Model file for the job. Use its own axes, mm. Face numbers are marked on the shaded views. A direction names the side the tool comes from. Coordinates: 2 decimals unless noted, no trailing zeros. Loops run counter-clockwise (first coordinate to the right, second up) from the corner with the lowest first, then second, coordinate; pieces in that order, holes last.
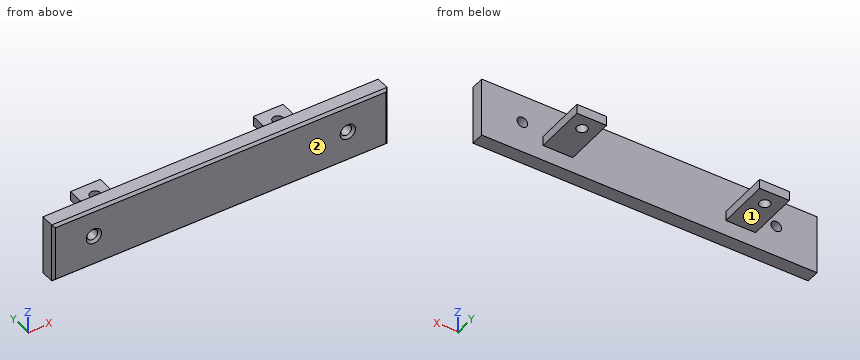
from build123d import *

# Parameters (mm, degrees)
SKETCH059_W             = 140
SKETCH059_H             = 25
SKETCH059_R             = 2.2
PAD026_DEPTH            = 6.5
SKETCH060_W             = 12.4
SKETCH060_H             = 4
PAD027_DEPTH            = 21.5
SKETCH061_R             = 2.2
POCKET032_DEPTH         = 10.609
CHAMFER024_SIZE         = 1
BODY013_ROLL_ANGLE      = 90
BODY013_PLACEMENT_ANGLE = 180


with BuildPart() as part:
    # Sketch059 → Pad026 (new body)
    with BuildSketch(Plane.XY):
        Rectangle(SKETCH059_W, SKETCH059_H)
        with Locations((-53, 0.726)):
            Circle(SKETCH059_R, mode=Mode.SUBTRACT)
        with Locations((53, 0.726)):
            Circle(SKETCH059_R, mode=Mode.SUBTRACT)
    extrude(amount=PAD026_DEPTH)

    # Sketch060 (on Face8 of Pad026) → Pad027 (join)
    with BuildSketch(Plane.XY.offset(6.5)):
        with Locations((-38.154, -3.892)):
            Rectangle(SKETCH060_W, SKETCH060_H)
        with Locations((38.154, -3.892)):
            Rectangle(SKETCH060_W, SKETCH060_H)
    extrude(amount=PAD027_DEPTH)

    # Sketch061 (on Face12 of Pad027) → Pocket032 (cut, through all)
    with BuildSketch(Plane(origin=(0, -1.892, 0), x_dir=(-1, 0, 0), z_dir=(0, 1, 0))):
        with Locations((-38.154, 21.8)):
            Circle(SKETCH061_R)
        with Locations((38.154, 21.8)):
            Circle(SKETCH061_R)
    extrude(amount=-POCKET032_DEPTH, mode=Mode.SUBTRACT)

    # Chamfer024
    chamfer024_edges = [part.edges().sort_by_distance(p)[0] for p in [
        (0, 12.5, 0),
        (70, 0, 0),
        (0, -12.5, 0),
        (-70, 0, 0),
        (50.8, 0.726, 0),
        (-55.2, 0.726, 0),
    ]]
    chamfer(chamfer024_edges, length=CHAMFER024_SIZE)


with BuildPart() as part_1:
    # Body013 roll: moved
    add(part.part.rotate(Axis((0, 0, 0), (1, 0, 0)), BODY013_ROLL_ANGLE))


with BuildPart() as part_2:
    # Body013 placement: moved
    add(part_1.part.moved(Location((0, -145.15, 0))).rotate(Axis((0, -145.15, 0), (0, 0, 1)), BODY013_PLACEMENT_ANGLE))


solid = part_2.part
Q1. Slice it at D-D (x = -19). List the corners of the cut face in (y, z), and give its area (4 significant figures).
Answers:
outline: (-145.15, -11.5) - (-144.15, -12.5) - (-138.65, -12.5) - (-138.65, 12.5) - (-144.15, 12.5) - (-145.15, 11.5) - close
area: 161.5 mm2
Q2. Which spindle directions (+Z, -Z, +X, -X, +Y, -Y) get a long thin tool onto all of the face, cutting with end or side? Do the marked faces 1 and 2. Say none if no direction does.
Answers:
face 1: -Z, +X, -X, +Y
face 2: +Z, -Z, +X, -X, -Y
Q3. Drill centre lines: line 1 (X direction, y = -123.35, z = -3.6); line 2 (Z direction, x = -53, y = -140.15); line 3 (X direction, y = -136, z = -2.75). Where is each one in solid material? Low to high.
Answers:
line 1: x = -44.35 to -40.35, -35.95 to -31.95, 31.95 to 35.95, 40.35 to 44.35
line 2: z = -12.5 to -1.47, 2.93 to 12.5
line 3: x = -44.35 to -31.95, 31.95 to 44.35
Q4. Flat gauge pins, fed straight in: P1, Ø7, axis at x = 53, z = 0.726, coming from the +Y side; P2, Ø1.5, axis at y = -133.5, z = 0, coming from the -X side; P3, Ø6, axis at x = 41, y = -128, coming from the -Z side; P4, Ø6, axis at x = -32, z = -7.5, coming from the +Y side. Where does each tip first touch, or does it go through?
Answers:
P1: stops at y = -138.65
P2: passes through
P3: stops at z = -5.89
P4: stops at y = -117.15
Q5. Slice it at B-B (y = -123.35). List the corners of the cut face in (x, z).
Answers:
outline: (-44.35, -5.89) - (-40.35, -5.89) - (-40.35, -1.89) - (-44.35, -1.89) - close; (-35.95, -5.89) - (-31.95, -5.89) - (-31.95, -1.89) - (-35.95, -1.89) - close; (31.95, -5.89) - (35.95, -5.89) - (35.95, -1.89) - (31.95, -1.89) - close; (40.35, -5.89) - (44.35, -5.89) - (44.35, -1.89) - (40.35, -1.89) - close
Q6. Slice it at C-C (y = -133). List the corners of the cut face in (x, z).
Answers:
outline: (-44.35, -5.89) - (-31.95, -5.89) - (-31.95, -1.89) - (-44.35, -1.89) - close; (31.95, -5.89) - (44.35, -5.89) - (44.35, -1.89) - (31.95, -1.89) - close
Q7. Slice it at A-A (x = 53). List the corners of the cut face in (y, z), and give its area (3 significant figures).
Answers:
outline: (-145.15, -11.5) - (-144.15, -12.5) - (-138.65, -12.5) - (-138.65, -1.47) - (-144.15, -1.47) - (-145.15, -2.47) - close; (-145.15, 3.93) - (-144.15, 2.93) - (-138.65, 2.93) - (-138.65, 12.5) - (-144.15, 12.5) - (-145.15, 11.5) - close
area: 132 mm2
